Part print with two shaded views. Sizes in mm from the minimum x, y, z corner. A direction names the side the tool comes from. Round coordinates to 2 decimals unless told otherwise and drop trailing zeros. Write each loop counter-clockwise with the first axis right and the second up, starting at its lowest first coordinate (ties: lowest second). Pieces come first, ordered by that corner, then holes. Notation, with made-up numbers: (57.5, 43) -> (94.5, 43) arc R25 ccw to (94.5, 80) -> close; hole circle Ø2 at (11.5, 16.25). An arc over 180 degrees is marked (long way). Return JSON: item names as keys, results as strings. Group by question number.
(1) Tool access for the marked faces 1 and 2: list every direction of +Z, -Z, +X, -X, +Y, -Y with a clear straight run to the whole face (end or side of a thin tool).
(2) Saw through at C-C (x = 38.1). List the corners of the cut face in (y, z).
(3) Saw through at A-A (x = 6.35). List the corners of the cut face in (y, z), plus the area to 3 significant figures.
(4) Drill centre lines: L1, parallel to Y at x = 38.1, z = 7; L2, parallel to Z at x = 6.35, y = 47; L3, parallel to X at y = 23, z = 22.5. Where is each one in solid material? Low to high. Write a range as from..to.
(5) Mould opens along Y. For the marked faces 3, 4 and 5 say: +Y half, -Y half, draft (parallel to the pull), parting line (faces both ways), or undercut.
(6) Saw through at B-B (z = 12.7). List the corners of the cut face in (x, y), plus the area to 3 significant figures.
(7) Saw through at D-D (z = 6). List the corners of the cut face in (x, y), plus the area to 3 significant figures.
(8) Drop flat-ended pins along their axis: pin 1 Ø4 at (x, z) = (10.5, 5.5) entering from -Y; pin 2 Ø12.5 at (y, z) = (20.5, 9) entering from +X. Give the stop position or say it passes through.
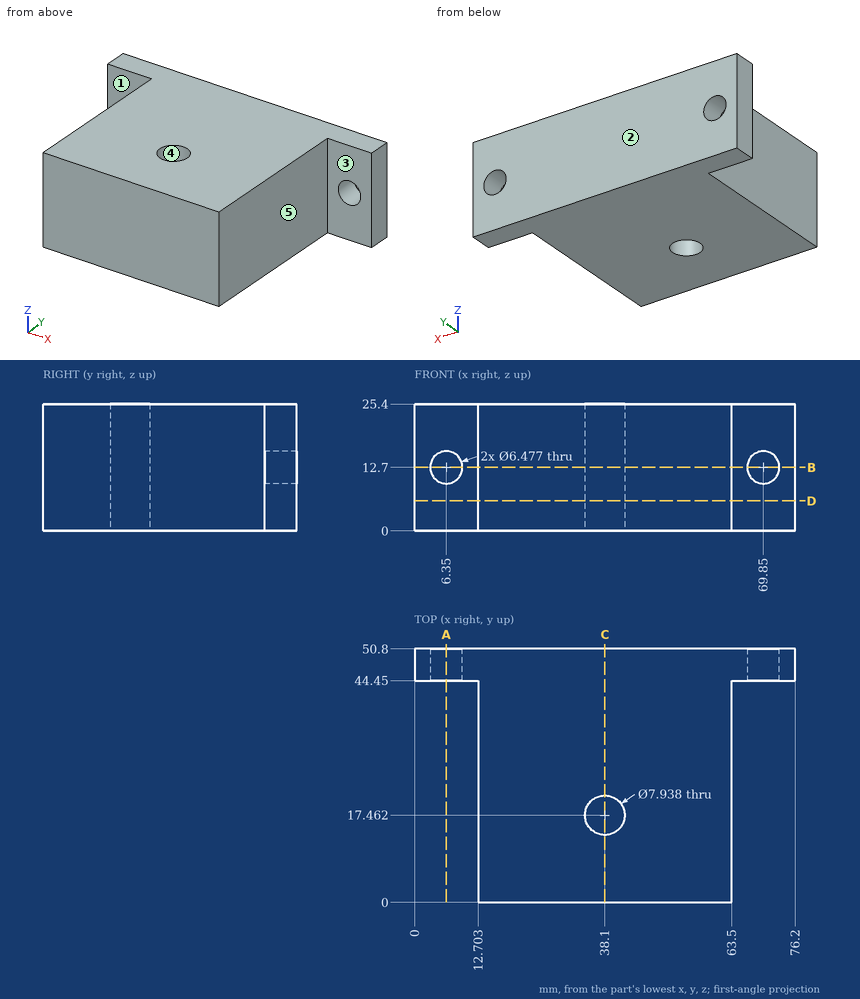
Computed values:
{
 "1": {"face 1": "+Z, -Z, -X, -Y", "face 2": "+Z, -Z, +X, -X, +Y"},
 "2": {"outline": "(0, 0) -> (13.49, 0) -> (13.49, 25.4) -> (0, 25.4) -> close; (21.43, 0) -> (50.8, 0) -> (50.8, 25.4) -> (21.43, 25.4) -> close"},
 "3": {"outline": "(44.45, 0) -> (50.8, 0) -> (50.8, 9.46) -> (44.45, 9.46) -> close; (44.45, 15.94) -> (50.8, 15.94) -> (50.8, 25.4) -> (44.45, 25.4) -> close", "area": "120 mm2"},
 "4": {"L1": "0..13.49, 21.43..50.8", "L2": "0..9.46, 15.94..25.4", "L3": "12.7..63.5"},
 "5": {"face 3": "-Y half", "face 4": "undercut", "face 5": "draft"},
 "6": {"outline": "(0, 44.45) -> (3.11, 44.45) -> (3.11, 50.8) -> (0, 50.8) -> close; (9.59, 44.45) -> (12.7, 44.45) -> (12.7, 0) -> (63.5, 0) -> (63.5, 44.45) -> (66.61, 44.45) -> (66.61, 50.8) -> (9.59, 50.8) -> close; (73.09, 44.45) -> (76.2, 44.45) -> (76.2, 50.8) -> (73.09, 50.8) -> close; hole circle Ø7.94 at (38.1, 17.46)", "area": "2,610 mm2"},
 "7": {"outline": "(0, 44.45) -> (12.7, 44.45) -> (12.7, 0) -> (63.5, 0) -> (63.5, 44.45) -> (76.2, 44.45) -> (76.2, 50.8) -> (0, 50.8) -> close; hole circle Ø7.94 at (38.1, 17.46)", "area": "2,690 mm2"},
 "8": {"pin 1": "y = 44.45", "pin 2": "x = 63.5"}
}
